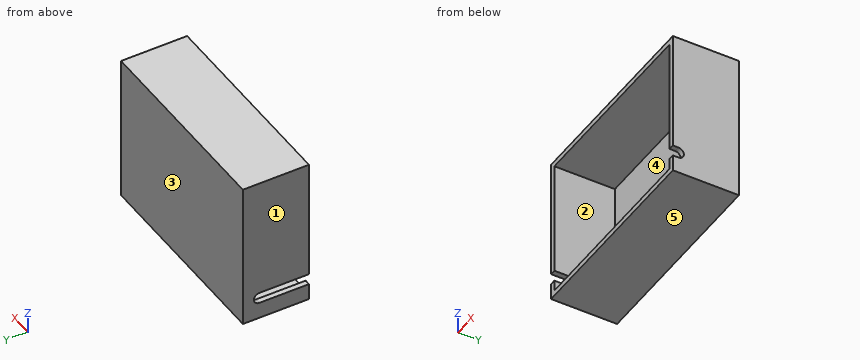
from build123d import *

# Parameters (mm, degrees)
F0_W     = 185
F0_H     = 135
F1_DEPTH = 60
F2_W     = 175
F2_H     = 125
F3_DEPTH = 55
F5_DEPTH = 25
F7_DEPTH = 25


with BuildPart() as f1:
    # F0 (on Front) → F1 (new body)
    with BuildSketch(Plane.XZ):
        with Locations((92.5, 67.5)):
            Rectangle(F0_W, F0_H)
    extrude(amount=F1_DEPTH)

    # F2 (on face) → F3 (cut)
    with BuildSketch(Plane.XZ.offset(60)):
        with Locations((92.5, 67.5)):
            Rectangle(F2_W, F2_H)
    extrude(amount=-F3_DEPTH, mode=Mode.SUBTRACT)

    # F4 (on face) → F5 (cut)
    with BuildSketch(Plane.YZ.offset(185)):
        with BuildLine():
            ThreePointArc((-55, 15), (-51.4644660941, 16.4644660941), (-50, 20))
            ThreePointArc((-50, 20), (-51.4644660941, 23.5355339059), (-55, 25))
            Line((-55, 25), (-55, 15))
        make_face()
        with BuildLine():
            Line((-55, 15), (-55, 25))
            ThreePointArc((-55, 25), (-60, 20), (-55, 15))
        make_face()
        with BuildLine():
            ThreePointArc((-55, 15), (-60, 20), (-55, 25))
            Line((-55, 25), (-65, 25))
            Line((-65, 25), (-65, 15))
            Line((-65, 15), (-55, 15))
        make_face()
    extrude(amount=-F5_DEPTH, mode=Mode.SUBTRACT)

    # F6 (on face) → F7 (cut)
    with BuildSketch(Plane(origin=(0, 0, 0), x_dir=(0, -1, 0), z_dir=(-1, 0, 0))):
        with BuildLine():
            Line((60, 15), (60, 25))
            Line((60, 25), (15, 25))
            ThreePointArc((15, 25), (18.5355339059, 23.5355339059), (20, 20))
            ThreePointArc((20, 20), (18.5355339059, 16.4644660941), (15, 15))
            Line((15, 15), (60, 15))
        make_face()
        with BuildLine():
            ThreePointArc((20, 20), (18.5355339059, 23.5355339059), (15, 25))
            Line((15, 25), (15, 15))
            ThreePointArc((15, 15), (18.5355339059, 16.4644660941), (20, 20))
        make_face()
        with BuildLine():
            Line((15, 15), (15, 25))
            ThreePointArc((15, 25), (10, 20), (15, 15))
        make_face()
    extrude(amount=-F7_DEPTH, mode=Mode.SUBTRACT)


solid = f1.part
Geometry: final body of the model. Coordinates: model frame, mm. Face numbers are marked on the shaded views. A direction names the side the tool comes from. Give positions to 0.01 mm unless a question says otherwise; leave off trailing zeros. Order: outer loops, then holes, each group sorted by start corner. A loop starts at its lowest first (then second) coordinate and runs counter-clockwise, first axis right, second up. Notation, with made-up numbers: (69, -13) - (93, -13) arc R12 ccw to (93, 3) - close; hole circle Ø7 at (68.25, 89). An arc over 180 degrees is marked (long way). Use CSV: the item, a comma, the result in double quotes.
1. Mould query, pull axis X, two halves, no side actions, for the marked faces 1, 2 and 3. Classes: +X half, -X half, draft (parallel to the pull), parting line (faces both ways), or undercut.
Answers below:
face 1,"-X half"
face 2,"undercut"
face 3,"draft"
2. Section query A-A (y = -33). Output: boundary loops of the cut face in (x, z).
Answers below:
outline,"(0, 0) - (185, 0) - (185, 135) - (0, 135) - (0, 25) - (5, 25) - (5, 130) - (180, 130) - (180, 5) - (5, 5) - (5, 15) - (0, 15) - close"
3. Section query C-C (z = 98). Output: boundary loops of the cut face in (x, y).
Answers below:
outline,"(0, -60) - (5, -60) - (5, -5) - (180, -5) - (180, -60) - (185, -60) - (185, 0) - (0, 0) - close"
4. Contact query for a flat-ended pin moving along its axis: pin 1 (2 mm diameter, centred on x = 76, z = 63.5, fed in from -Y). Output: stop coordinate, or through.
Answers below:
pin 1,"y = -5"
5. Access query for the marked faces 4 and 5. Directions: +Z, -Z, +X, -X, +Y, -Y. A direction counts if a zero-diameter tool reaches every point of the face in a straight line with its end or side. Return the directions, or none.
Answers below:
face 4,"-Y"
face 5,"-Z, +X, -X, +Y, -Y"
6. Section query B-B (x = 102.5). Output: boundary loops of the cut face in (y, z).
Answers below:
outline,"(-60, 0) - (0, 0) - (0, 135) - (-60, 135) - (-60, 130) - (-5, 130) - (-5, 5) - (-60, 5) - close"
7. Material intervals for line 1 along Z through (x, y) = (58, -37.5); line 2 along X through (y, z) = (-55, 8); line 3 along Y through (x, z) = (72, 104.5), sorted ascending. Write a range as from..to.
Answers below:
line 1,"0..5, 130..135"
line 2,"0..5, 180..185"
line 3,"-5..0"
